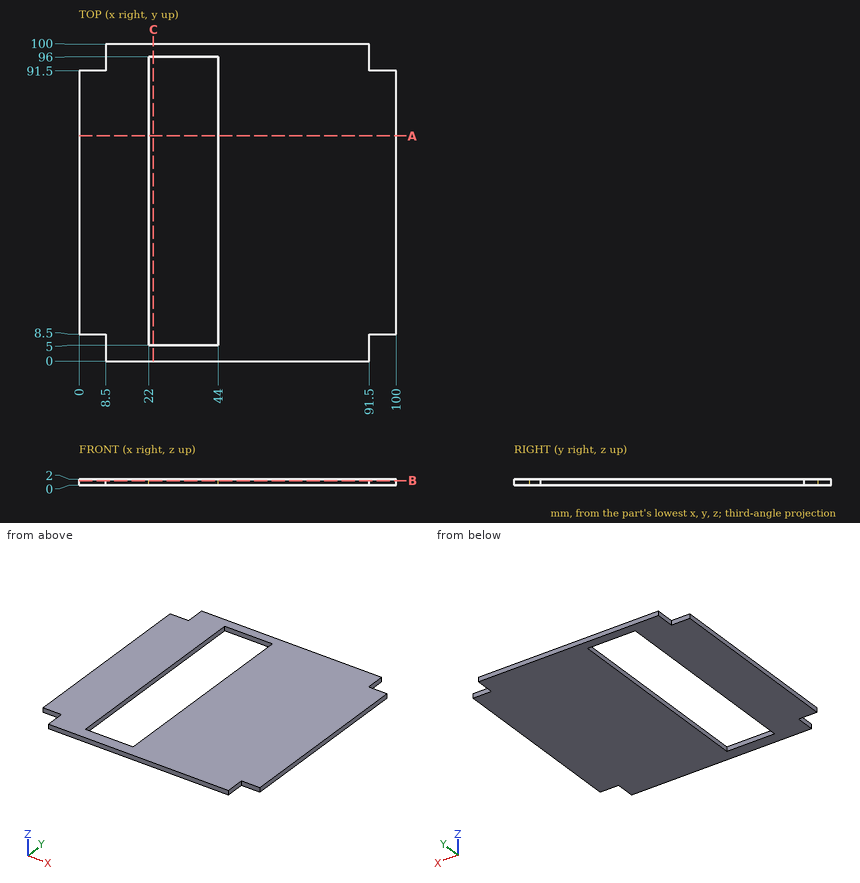
Design review of the part shown in the three views and the two pictorial views. Dimensions are in mm from the part's minimum x, y and z. Round coordinates to 2 decimals unless told otherwise and drop trailing zeros. Write each loop counter-clockwise with the first axis right and the second up, starting at its lowest first coordinate (ties: lowest second). Pieces come first, ordered by that corner, then holes.
Item 1: Wall thickness on L1, parallel to Y at x = 37, z = 0.6; L2, parallel to X at y = 20, z = 1.9; L3, parallel to Y at x = 7, z = 1.5: over which ranges is each line inside the solid? List them lowest first.
Item 2: Consider section B-B on z = 1.5. Give the boundary of the cut face in (x, y), and give its area (3 significant figures).
Item 3: Consider section A-A on y = 71. Give the boundary of the cut face in (x, z).
Item 4: For pin 1 Ø1 at (y, z) = (52.5, 0.5) entering from -X; pin 2 Ø10 at (x, y) = (38, 56) entering from -Z; pin 3 Ø0.6 at (y, z) = (3.5, 1) entering from +X; pin 4 Ø0.6 at (x, z) = (94, 0.5) entering from -Y, all flat-tipped, find the tip position at first contact; note any pin that passes through.
Item 5: Consider section C-C on x = 23.5. Give the boundary of the cut face in (y, z).
Check values:
1. L1: y = 0 to 5, 96 to 100
1. L2: x = 0 to 22, 44 to 100
1. L3: y = 8.5 to 91.5
2. outline: (0, 8.5) - (8.5, 8.5) - (8.5, 0) - (91.5, 0) - (91.5, 8.5) - (100, 8.5) - (100, 91.5) - (91.5, 91.5) - (91.5, 100) - (8.5, 100) - (8.5, 91.5) - (0, 91.5) - close; hole (22, 5) - (44, 5) - (44, 96) - (22, 96) - close
2. area: 7,710 mm2
3. outline: (0, 0) - (22, 0) - (22, 2) - (0, 2) - close; (44, 0) - (100, 0) - (100, 2) - (44, 2) - close
4. pin 1: stops at x = 0
4. pin 2: passes through
4. pin 3: stops at x = 91.5
4. pin 4: stops at y = 8.5
5. outline: (0, 0) - (5, 0) - (5, 2) - (0, 2) - close; (96, 0) - (100, 0) - (100, 2) - (96, 2) - close
